The model under review builds one solid part; all positions refer to its coordinate system, in mm. Face numbers are marked on the shaded views. A direction names the side the tool comes from. Coordinates: 2 decimals unless noted, no trailing zeros. Loops run counter-clockwise (first coordinate to the right, second up) from the corner with the lowest first, then second, coordinate; pieces in that order, holes last. Notation, with made-up numbers: M -2,-9.5 L 5,-9.5 A19 ccw 5,0.5 Z; hole C 35.25,34 d1. An arc over 180 degrees is marked long. Use CSV: the item, a comma, the result in double quotes. Start each with the question number.
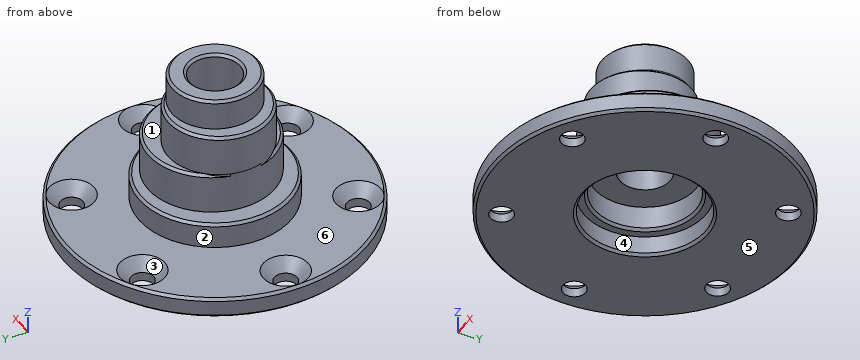
from build123d import *

# Parameters (mm, degrees)
SKETCH1_R                                    = 30
BOSS_EXTRUDE1_DEPTH                          = 4
CSK_FOR_M4_HEX_SOCKET_COUNTERSUNK_CA_2_COUNT = 2
CSK_FOR_M4_HEX_SOCKET_COUNTERSUNK_CA_2_PITCH = 25
CSK_FOR_M4_HEX_SOCKET_COUNTERSUNK_CA_3_COUNT = 2
CSK_FOR_M4_HEX_SOCKET_COUNTERSUNK_CA_3_PITCH = 43.301270189
CSK_FOR_M4_HEX_SOCKET_COUNTERSUNK_CA_4_COUNT = 2
CSK_FOR_M4_HEX_SOCKET_COUNTERSUNK_CA_4_PITCH = 43.301270189
CSK_FOR_M4_HEX_SOCKET_COUNTERSUNK_CA_5_COUNT = 2
CSK_FOR_M4_HEX_SOCKET_COUNTERSUNK_CA_5_PITCH = 50
CSK_FOR_M4_HEX_SOCKET_COUNTERSUNK_CA_6_COUNT = 2
CSK_FOR_M4_HEX_SOCKET_COUNTERSUNK_CA_6_PITCH = 25
SKETCH2_R                                    = 15.05
SKETCH2_R_2                                  = 10.05
BOSS_EXTRUDE3_DEPTH                          = 5
SKETCH5_R                                    = 12
CUT_EXTRUDE2_DEPTH                           = 4
SKETCH6_R                                    = 12.55
BOSS_EXTRUDE4_DEPTH                          = 8
SKETCH7_R                                    = 10.05
BOSS_EXTRUDE5_DEPTH                          = 8
SKETCH8_R                                    = 8.55
BOSS_EXTRUDE6_DEPTH                          = 6
SKETCH9_R                                    = 5
CUT_EXTRUDE3_DEPTH                           = 30
CHAMFER1_SIZE                                = 0.5


with BuildPart() as part:
    # Sketch1 → Boss-Extrude1 (new body)
    with BuildSketch(Plane.XY):
        Circle(SKETCH1_R)
    extrude(amount=BOSS_EXTRUDE1_DEPTH)

    # Sketch3 → CSK for M4 Hex Socket Countersunk Cap Screw1 (revolve, cut)
    with BuildSketch(Plane(origin=(-12.5, 21.650635095, 4), x_dir=(0, -1, 0), z_dir=(1, 0, 0))):
        Polygon((0, 0), (0, 4), (2.25, 4), (2.25, 2.23), (4.48, 0), align=None)
    csk_for_m4_hex_socket_countersunk_cap_sc = revolve(axis=Axis((-12.5, 21.650635095, 10.35), (0, 0, -1)), mode=Mode.SUBTRACT)

    # CSK for M4 Hex Socket Countersunk Ca 2: CSK for M4 Hex Socket Countersunk Cap Screw1 ×2
    with Locations(*[(i * CSK_FOR_M4_HEX_SOCKET_COUNTERSUNK_CA_2_PITCH, 0, 0) for i in range(1, CSK_FOR_M4_HEX_SOCKET_COUNTERSUNK_CA_2_COUNT)]):
        add(csk_for_m4_hex_socket_countersunk_cap_sc, mode=Mode.SUBTRACT)

    # CSK for M4 Hex Socket Countersunk Ca 3: CSK for M4 Hex Socket Countersunk Cap Screw1 ×2
    with Locations(*[Vector(0.8660254037844606, -0.4999999999999621, 0) * (i * CSK_FOR_M4_HEX_SOCKET_COUNTERSUNK_CA_3_PITCH) for i in range(1, CSK_FOR_M4_HEX_SOCKET_COUNTERSUNK_CA_3_COUNT)]):
        add(csk_for_m4_hex_socket_countersunk_cap_sc, mode=Mode.SUBTRACT)

    # CSK for M4 Hex Socket Countersunk Ca 4: CSK for M4 Hex Socket Countersunk Cap Screw1 ×2
    with Locations(*[(0, -i * CSK_FOR_M4_HEX_SOCKET_COUNTERSUNK_CA_4_PITCH, 0) for i in range(1, CSK_FOR_M4_HEX_SOCKET_COUNTERSUNK_CA_4_COUNT)]):
        add(csk_for_m4_hex_socket_countersunk_cap_sc, mode=Mode.SUBTRACT)

    # CSK for M4 Hex Socket Countersunk Ca 5: CSK for M4 Hex Socket Countersunk Cap Screw1 ×2
    with Locations(*[Vector(0.5000000000000379, -0.8660254037844168, 0) * (i * CSK_FOR_M4_HEX_SOCKET_COUNTERSUNK_CA_5_PITCH) for i in range(1, CSK_FOR_M4_HEX_SOCKET_COUNTERSUNK_CA_5_COUNT)]):
        add(csk_for_m4_hex_socket_countersunk_cap_sc, mode=Mode.SUBTRACT)

    # CSK for M4 Hex Socket Countersunk Ca 6: CSK for M4 Hex Socket Countersunk Cap Screw1 ×2
    with Locations(*[Vector(-0.49999999999996236, -0.8660254037844605, 0) * (i * CSK_FOR_M4_HEX_SOCKET_COUNTERSUNK_CA_6_PITCH) for i in range(1, CSK_FOR_M4_HEX_SOCKET_COUNTERSUNK_CA_6_COUNT)]):
        add(csk_for_m4_hex_socket_countersunk_cap_sc, mode=Mode.SUBTRACT)

    # Sketch2 → Boss-Extrude3 (add)
    with BuildSketch(Plane.XY.offset(4)):
        Circle(SKETCH2_R)
        Circle(SKETCH2_R_2, mode=Mode.SUBTRACT)
    extrude(amount=BOSS_EXTRUDE3_DEPTH)

    # Sketch5 → Cut-Extrude2 (cut)
    with BuildSketch(Plane(origin=(0, 0, 0), x_dir=(-1, 0, 0), z_dir=(0, 0, -1))):
        Circle(SKETCH5_R)
    extrude(amount=-CUT_EXTRUDE2_DEPTH, mode=Mode.SUBTRACT)

    # Sketch6 → Boss-Extrude4 (add)
    with BuildSketch(Plane.XY.offset(9)):
        with Locations((1.3, 0)):
            Circle(SKETCH6_R)
    extrude(amount=BOSS_EXTRUDE4_DEPTH)

    # Sketch7 → Boss-Extrude5 (add)
    with BuildSketch(Plane.XY.offset(17)):
        with Locations(Location((-1.3, 0, 0), (0, 0, 162.13454876))):
            Circle(SKETCH7_R)
    extrude(amount=BOSS_EXTRUDE5_DEPTH)

    # Sketch8 → Boss-Extrude6 (add)
    with BuildSketch(Plane.XY.offset(25)):
        Circle(SKETCH8_R)
    extrude(amount=BOSS_EXTRUDE6_DEPTH)

    # Sketch9 → Cut-Extrude3 (cut)
    with BuildSketch(Plane.XY.offset(31)):
        Circle(SKETCH9_R)
    extrude(amount=-CUT_EXTRUDE3_DEPTH, mode=Mode.SUBTRACT)

    # Chamfer1
    # the kernel refuses this chamfer: 0.5 mm, written as the material it takes off along each edge
    with BuildSketch(Plane(origin=(0, 0, 0), x_dir=(1, 0, 0), z_dir=(0, -1, 0))) as chamfer1_piece_1:
        Polygon((30, CHAMFER1_SIZE), (30 - CHAMFER1_SIZE, 0), (30, 0), align=None)
    revolve(axis=Axis((0, 0, 0), (0, 0, 1)), mode=Mode.SUBTRACT)
    with BuildSketch(Plane(origin=(0, 0, 9), x_dir=(1, 0, 0), z_dir=(0, -1, 0))) as chamfer1_piece_2:
        Polygon((15.05, -CHAMFER1_SIZE), (15.05 - CHAMFER1_SIZE, 0), (15.05, 0), align=None)
    revolve(axis=Axis((0, 0, 9), (0, 0, 1)), mode=Mode.SUBTRACT)
    with BuildSketch(Plane(origin=(0, 0, 4), x_dir=(1, 0, 0), z_dir=(0, -1, 0))) as chamfer1_piece_3:
        Polygon((30, -CHAMFER1_SIZE), (30 - CHAMFER1_SIZE, 0), (30, 0), align=None)
    revolve(axis=Axis((0, 0, 4), (0, 0, 1)), mode=Mode.SUBTRACT)
    with BuildSketch(Plane(origin=(0, 0, 4), x_dir=(1, 0, 0), z_dir=(0, -1, 0))) as chamfer1_piece_4:
        Polygon((10.05 + CHAMFER1_SIZE, 0), (10.05, CHAMFER1_SIZE), (10.05, 0), align=None)
    revolve(axis=Axis((0, 0, 4), (0, 0, 1)), mode=Mode.SUBTRACT)
    with BuildSketch(Plane(origin=(0, 0, 0), x_dir=(-1, 0, 0), z_dir=(0, -1, 0))) as chamfer1_piece_5:
        Polygon((12 + CHAMFER1_SIZE, 0), (12, -CHAMFER1_SIZE), (12, 0), align=None)
    revolve(axis=Axis((0, 0, 0), (0, 0, -1)), mode=Mode.SUBTRACT)
    with BuildSketch(Plane(origin=(1.3, 0, 17), x_dir=(-0.9894169628260336, -0.1451002194075096, 0), z_dir=(-0.1451002194075096, 0.9894169628260336, 0))) as chamfer1_piece_6_section:
        Polygon((12.55, -CHAMFER1_SIZE), (12.55 - CHAMFER1_SIZE, 0), (12.55, 0), align=None)
    chamfer1_piece_6 = revolve(axis=Axis((1.3, 0, 17), (0, 0, 1)), revolution_arc=171.656917286, mode=Mode.PRIVATE)
    chamfer1_piece_6 = chamfer1_piece_6 - Plane(origin=(-1.3, 0, 16.761451234), x_dir=(-0.9517795637185023, 0.3067827604149514, 0), z_dir=(0, 0, -1)) * Cylinder(10.05, 51, mode=Mode.PRIVATE)
    add(chamfer1_piece_6, mode=Mode.SUBTRACT)
    with BuildSketch(Plane(origin=(-1.3, 0, 25), x_dir=(-0.9517795637185023, 0.3067827604149514, 0), z_dir=(0.3067827604149514, 0.9517795637185023, 0))) as chamfer1_piece_7_section:
        Polygon((10.05, -CHAMFER1_SIZE), (10.05 - CHAMFER1_SIZE, 0), (10.05, 0), align=None)
    chamfer1_piece_7 = revolve(axis=Axis((-1.3, 0, 25), (0, 0, 1)), mode=Mode.PRIVATE)
    chamfer1_piece_7 = chamfer1_piece_7 - Plane(origin=(0, 0, 24.76381896), x_dir=(1, 0, 0), z_dir=(0, 0, -1)) * Cylinder(8.55, 41, mode=Mode.PRIVATE)
    add(chamfer1_piece_7, mode=Mode.SUBTRACT)
    with BuildSketch(Plane(origin=(0, 0, 31), x_dir=(1, 0, 0), z_dir=(0, -1, 0))) as chamfer1_piece_8:
        Polygon((8.55 - CHAMFER1_SIZE, 0), (8.55, -CHAMFER1_SIZE), (8.55, 0), align=None)
    revolve(axis=Axis((0, 0, 31), (0, 0, 1)), mode=Mode.SUBTRACT)
    with BuildSketch(Plane(origin=(0, 0, 31), x_dir=(1, 0, 0), z_dir=(0, -1, 0))) as chamfer1_piece_9:
        Polygon((5, -CHAMFER1_SIZE), (5 + CHAMFER1_SIZE, 0), (5, 0), align=None)
    revolve(axis=Axis((0, 0, 31), (0, 0, 1)), mode=Mode.SUBTRACT)
    with BuildSketch(Plane(origin=(1.3, 0, 17), x_dir=(1, 0, 0), z_dir=(0, -1, 0))) as chamfer1_piece_10_section:
        Polygon((12.55, -CHAMFER1_SIZE), (12.55 - CHAMFER1_SIZE, 0), (12.55, 0), align=None)
    chamfer1_piece_10 = revolve(axis=Axis((1.3, 0, 17), (0, 0, 1)), revolution_arc=171.656917286, mode=Mode.PRIVATE)
    chamfer1_piece_10 = chamfer1_piece_10 - Plane(origin=(-1.3, 0, 16.761451234), x_dir=(-0.9517795637185023, 0.3067827604149514, 0), z_dir=(0, 0, -1)) * Cylinder(10.05, 51, mode=Mode.PRIVATE)
    add(chamfer1_piece_10, mode=Mode.SUBTRACT)


solid = part.part
1. Add section C-C (z = 26). Write out the cut boundary in (x, y).
2. Draft analysis for pull direction X (two halves, no side actions). For the marked faces 1, 2 and 3, state which applies: released by +X, released by -X, zero draft, split by the parting line, or undercut.
3. Add section B-B (y = 1.5). Give the number of separate pieces and of enclosed holes in the cut face, plus the area to 3 significant figures.
4. Insertion check: pin 1 Ø5 at (y, z) = (14.5, 20) entering from -X; pin 2 Ø11.5 at (x, y) = (0, 0) entering from +Z; pin 3 Ø16 at (x, y) = (0, 2.5) entering from -Z; pin 4 Ø12 at (y, z) = (12, 23.5) entering from +X. Each pin has a flat end and moves straight along its axis. Give the tip position at first contact, or say it passes through.
5. For the marked faces 4, 5 and 6, list the 3-axis set-ups (+Z, -Z, +X, -X, +Y, -Y) from which the entire face can be reached by the end or side of a thin tool; tool diameter is ignored.
6. To check wall thickness, follow line 1 along Y through (x, z) = (0, 3); line 2 along X through (y, z) = (-23, 2.5); line 3 along Y through (x, z) = (0, 6). State the ranges of each line that lie inside material, in increasing order.
7. Add section A-A (z = 14.5). Write out the cut boundary in (x, y), plus the area to 3 significant figures.
Solved:
1,outline,"C 0,0 d17.1; hole C 0,0 d10"
2,face 1,"zero draft"
2,face 2,"split by the parting line"
2,face 3,"undercut"
3,separate pieces,"4"
3,enclosed holes,"0"
3,area,"404 mm^2"
4,pin 1,"passes through"
4,pin 2,"stops at z = 31"
4,pin 3,"stops at z = 4.05"
4,pin 4,"stops at x = 6.76"
5,face 4,"-Z"
5,face 5,"-Z, +X, -X, +Y, -Y"
5,face 6,"+Z"
6,line 1,"y = -30 to -12, 12 to 30"
6,line 2,"x = -19.26 to -15.16, -9.84 to 9.84, 15.16 to 19.26"
6,line 3,"y = -15.05 to -10.05, 10.05 to 15.05"
7,outline,"C 1.3,0 d25.1; hole C 0,0 d10"
7,area,"416 mm^2"
